The figure shows three views and two pictorial views of one solid part (mm, origin at its lowest corner). Answer the questions. A direction names the side the tool comes from. Give positions to 0.01 mm unless a question says otherwise; leave off trailing zeros. Order: outer loops, then holes, each group sorted by start corner. A loop starts at its lowest first (then second) coordinate and runs counter-clockwise, first axis right, second up. Notation, with made-up numbers: M -26,-2 L -13,-2 A25 ccw -13,14 Z; hole C 56.25,-32 d9. An arc over 180 degrees is marked long. Answer as a JSON object with one key per item and string values. Group by question number.
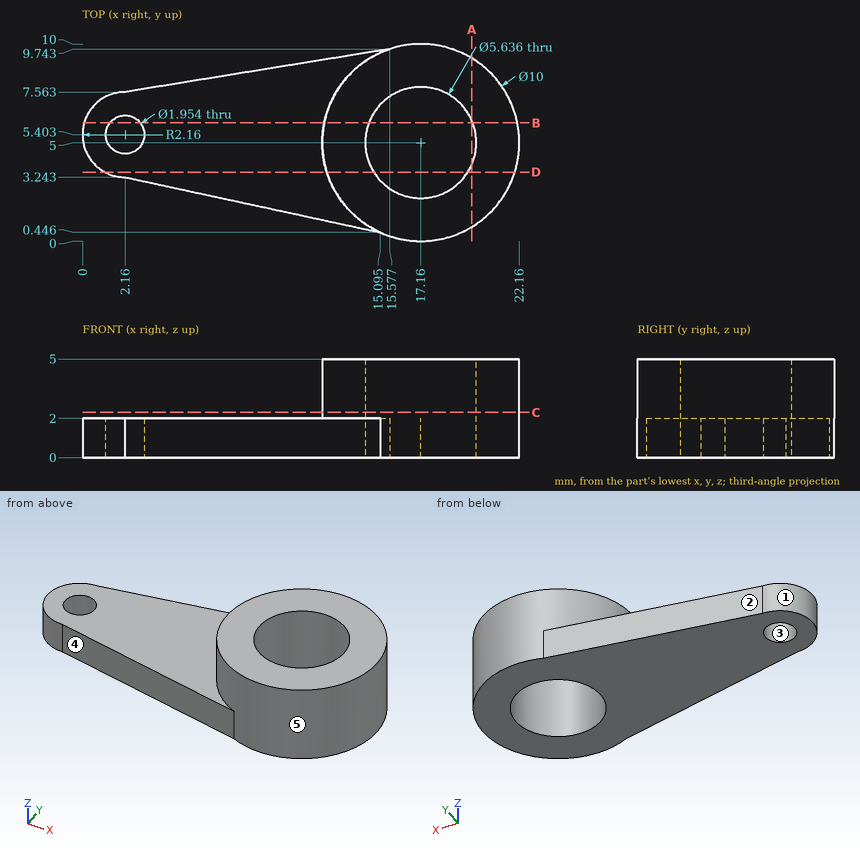
Item 1: Consider probe 1 along Z at (x, y) = (4.5, 5.75); probe 2 along X at (y, z) = (4.25, 1.2) (1 decimal); probe 3 along X at (y, z) = (7.5, 4.15) (1 decimal). Determine where each line is inside the solid, lowest interval first. Write a range as from..to.
Item 2: Section D-D (y = 3.5) is taken. Determine the outline of the cut face in (x, z) (1 decimal).
Item 3: Section C-C (z = 2.3) is taken. Determine the outline of the cut face in (x, y) (1 decimal).
Item 4: Section A-A (x = 19.75) is taken. Determine the outline of the cut face in (y, z).
Item 5: A tool of negligible diameter and unlimited length cuts with its end or side. For the marked faces 4 and 5, from which of +Z, -Z, +X, -X, +Y, -Y can it reach the whole face along a straight path? Write none if from no direction.
Item 6: Determine the mould class of the marked faces 1, 2 and 3 for opening direction Y: released by +Y, released by -Y, zero draft, split by the parting line, or undercut.
Item 7: Section B-B (y = 6) is taken. Determine the outline of the cut face in (x, z) (1 decimal).
Item 8: A flat-ended cylindrical pin translates along its axis: P1, Ø6, axis at x = 3.5, y = 1.5, coming from the +Z side. Find the tip coordinate at first contact, or state that the pin passes through.
Values found:
{
 "1": {"probe 1": "z = 0..2", "probe 2": "x = 0.3..14.4, 19.9..22.1", "probe 3": "x = 12.8..15.9, 18.5..21.5"},
 "2": {"outline": "M 1.1,0 L 14.8,0 L 14.8,5 L 12.4,5 L 12.4,2 L 1.1,2 Z; M 19.5,0 L 21.9,0 L 21.9,5 L 19.5,5 Z"},
 "3": {"outline": "C 17.2,5 d10; hole C 17.2,5 d5.6"},
 "4": {"outline": "M 0.72,0 L 3.89,0 L 3.89,5 L 0.72,5 Z; M 6.11,0 L 9.28,0 L 9.28,5 L 6.11,5 Z"},
 "5": {"face 4": "+Z, -Z, -X, -Y", "face 5": "+Z"},
 "6": {"face 1": "split by the parting line", "face 2": "released by +Y", "face 3": "undercut"},
 "7": {"outline": "M 0.1,0 L 1.4,0 L 1.4,2 L 0.1,2 Z; M 2.9,0 L 14.5,0 L 14.5,5 L 12.3,5 L 12.3,2 L 2.9,2 Z; M 19.8,0 L 22.1,0 L 22.1,5 L 19.8,5 Z"},
 "8": {"P1": "stops at z = 2"}
}
